```python
from build123d import *

# Parameters (mm, degrees)
SKETCH1_W           = 55.88
SKETCH1_H           = 45.72
BOSS_EXTRUDE1_DEPTH = 2.54
CUT_EXTRUDE1_REACH  = 4.54
SKETCH2_R           = 1.7
BOSS_EXTRUDE2_DEPTH = 2.21996
CUT_EXTRUDE2_DEPTH  = 2.21996
CUT_EXTRUDE3_REACH  = 6.76
SKETCH6_R           = 2.25
SKETCH7_W           = 7.62
SKETCH7_H           = 2.21996
CUT_EXTRUDE4_DEPTH  = 56.88
FILLET1_R           = 2.54


with BuildPart() as part:
    # Sketch1 → Boss-Extrude1 (new body)
    with BuildSketch(Plane(origin=(0, 0, 0), x_dir=(1, 0, 0), z_dir=(0, 1, 0))):
        with Locations((27.94, 22.86)):
            Rectangle(SKETCH1_W, SKETCH1_H)
    extrude(amount=BOSS_EXTRUDE1_DEPTH)

    # Sketch2 → Cut-Extrude1 (cut, up to next)
    with BuildSketch(Plane(origin=(0, 2.54, 0), x_dir=(1, 0, 0), z_dir=(0, 1, 0)), mode=Mode.PRIVATE) as cut_extrude1_sk1:
        with Locations((5.08, 40.64)):
            Circle(SKETCH2_R)
    cut_extrude1_tool1 = extrude(cut_extrude1_sk1.sketch, amount=-CUT_EXTRUDE1_REACH, mode=Mode.PRIVATE) & part.part
    add(cut_extrude1_tool1.solids().sort_by_distance((5.08, 2.54, -40.64))[0], mode=Mode.SUBTRACT)
    # Sketch2 → Cut-Extrude1 (cut, up to next)
    with BuildSketch(Plane(origin=(0, 2.54, 0), x_dir=(1, 0, 0), z_dir=(0, 1, 0)), mode=Mode.PRIVATE) as cut_extrude1_sk2:
        with Locations((50.8, 40.64)):
            Circle(SKETCH2_R)
    cut_extrude1_tool2 = extrude(cut_extrude1_sk2.sketch, amount=-CUT_EXTRUDE1_REACH, mode=Mode.PRIVATE) & part.part
    add(cut_extrude1_tool2.solids().sort_by_distance((50.8, 2.54, -40.64))[0], mode=Mode.SUBTRACT)
    # Sketch2 → Cut-Extrude1 (cut, up to next)
    with BuildSketch(Plane(origin=(0, 2.54, 0), x_dir=(1, 0, 0), z_dir=(0, 1, 0)), mode=Mode.PRIVATE) as cut_extrude1_sk3:
        with Locations((50.8, 5.08)):
            Circle(SKETCH2_R)
    cut_extrude1_tool3 = extrude(cut_extrude1_sk3.sketch, amount=-CUT_EXTRUDE1_REACH, mode=Mode.PRIVATE) & part.part
    add(cut_extrude1_tool3.solids().sort_by_distance((50.8, 2.54, -5.08))[0], mode=Mode.SUBTRACT)
    # Sketch2 → Cut-Extrude1 (cut, up to next)
    with BuildSketch(Plane(origin=(0, 2.54, 0), x_dir=(1, 0, 0), z_dir=(0, 1, 0)), mode=Mode.PRIVATE) as cut_extrude1_sk4:
        with Locations((5.08, 5.08)):
            Circle(SKETCH2_R)
    cut_extrude1_tool4 = extrude(cut_extrude1_sk4.sketch, amount=-CUT_EXTRUDE1_REACH, mode=Mode.PRIVATE) & part.part
    add(cut_extrude1_tool4.solids().sort_by_distance((5.08, 2.54, -5.08))[0], mode=Mode.SUBTRACT)

    # Sketch4 → Boss-Extrude2 (add)
    with BuildSketch(Plane(origin=(0, 2.54, 0), x_dir=(1, 0, 0), z_dir=(0, 1, 0))):
        Polygon((0, 30.48), (20.32, 45.72), (35.56, 45.72), (55.88, 30.48), (55.88, 15.24), (35.56, 0), (20.32, 0), (0, 15.24), align=None)
    extrude(amount=BOSS_EXTRUDE2_DEPTH)

    # Sketch5 → Cut-Extrude2 (cut)
    with BuildSketch(Plane.XZ):
        with BuildLine():
            Line((3.062941176, -18.986804383), (15.613529412, -8.335516435))
            ThreePointArc((15.613529412, -8.335516435), (27.94, -3.81), (40.266470588, -8.335516435))
            Line((40.266470588, -8.335516435), (52.817058824, -18.986804383))
            ThreePointArc((52.817058824, -18.986804383), (54.61, -22.86), (52.817058824, -26.733195617))
            Line((52.817058824, -26.733195617), (40.266470588, -37.384483565))
            ThreePointArc((40.266470588, -37.384483565), (27.94, -41.91), (15.613529412, -37.384483565))
            Line((15.613529412, -37.384483565), (3.062941176, -26.733195617))
            ThreePointArc((3.062941176, -26.733195617), (1.27, -22.86), (3.062941176, -18.986804383))
        make_face()
    extrude(amount=-CUT_EXTRUDE2_DEPTH, mode=Mode.SUBTRACT)

    # Sketch6 → Cut-Extrude3 (cut, up to next)
    with BuildSketch(Plane(origin=(0, 4.75996, 0), x_dir=(1, 0, 0), z_dir=(0, 1, 0)), mode=Mode.PRIVATE) as cut_extrude3_sk1:
        with Locations((6.35, 22.86)):
            Circle(SKETCH6_R)
    cut_extrude3_tool1 = extrude(cut_extrude3_sk1.sketch, amount=-CUT_EXTRUDE3_REACH, mode=Mode.PRIVATE) & part.part
    add(cut_extrude3_tool1.solids().sort_by_distance((6.35, 4.75996, -22.86))[0], mode=Mode.SUBTRACT)
    # Sketch6 → Cut-Extrude3 (cut, up to next)
    with BuildSketch(Plane(origin=(0, 4.75996, 0), x_dir=(1, 0, 0), z_dir=(0, 1, 0)), mode=Mode.PRIVATE) as cut_extrude3_sk2:
        with Locations((49.53, 22.86)):
            Circle(SKETCH6_R)
    cut_extrude3_tool2 = extrude(cut_extrude3_sk2.sketch, amount=-CUT_EXTRUDE3_REACH, mode=Mode.PRIVATE) & part.part
    add(cut_extrude3_tool2.solids().sort_by_distance((49.53, 4.75996, -22.86))[0], mode=Mode.SUBTRACT)

    # Sketch7 → Cut-Extrude4 (cut, through all)
    with BuildSketch(Plane.ZY):
        with Locations((-22.86, 1.10998)):
            Rectangle(SKETCH7_W, SKETCH7_H)
    extrude(amount=-CUT_EXTRUDE4_DEPTH, mode=Mode.SUBTRACT)

    # Fillet1
    fillet1_edges = [part.edges().sort_by_distance(p)[0] for p in [
        (0, 3.64998, -30.48),
        (0, 3.64998, -15.24),
        (20.32, 3.64998, 0),
        (35.56, 3.64998, 0),
        (55.88, 3.64998, -15.24),
        (55.88, 3.64998, -30.48),
        (35.56, 3.64998, -45.72),
        (20.32, 3.64998, -45.72),
    ]]
    fillet(fillet1_edges, radius=FILLET1_R)


solid = part.part
```
The listing builds one solid part. Answer for the finished solid, in the listing's coordinates (mm). A direction names the side the tool comes from. Coordinates: 2 decimals unless noted, no trailing zeros. Loops run counter-clockwise (first coordinate to the right, second up) from the corner with the lowest first, then second, coordinate; pieces in that order, holes last. Notation, with made-up numbers: (19, -1.5) -> (25, -1.5) arc R19 cw to (25, 30.5) -> close; hole circle Ø6 at (16, 61). An arc over 180 degrees is marked (long way). Return JSON: item names as keys, results as strings. Group by question number.
(1) A cutting plane is placed at A-A on y = 0.95. Write down the section's boundary in (x, z).
(2) A cutting plane is placed at B-B on z = -22.86. Write down the section's boundary in (x, y), and give its area (3 significant figures).
(3) Which of the six approach directions +Z, -Z, +X, -X, +Y, -Y give full straight-line access (tool end or side, diameter ignored) to faces 5 (the flat face through (50, 2.54, -7)), 6 (the flat face through (46.63, 1.094, -31.984)), 7 (the flat face through (8, 2.54, -41)), 8 (the flat face through (1, 1, -26.67)), 9 (the cylindrical face through (6.06, 3.51, -25.09))?
(4) Determine the mould class of faces 1 (the cylindrical face through (3.83, 1.29, -41.79)), 2 (the cylindrical face through (20.353, 3.666, -0.134)), 3 (the flat face through (48, 2.54, -41)), 4 (the flat face through (45.68, 3.63, -7.59)) for opening direction X: released by +X, released by -X, zero draft, split by the parting line, or undercut.
(5) Given pin 1 Ø4 at (x, z) = (5.08, -5.08) entering from +Y; pin 2 Ø5 at (x, z) = (6.35, -22.86) entering from -Y; pin 3 Ø2 at (x, z) = (50.8, -5.08) entering from +Y, each flat-ended and moving along its own axis, determine where each tip first touches the part or whether it passes through.
(6) Find the intervals of material crossed by probe 1 along X at (y, z) = (2.9, -22.86); probe 2 along Z at (x, y) = (5.08, 1.9) (3 decimals); probe 3 along X at (y, z) = (1, -40), in increasing order. Write a range as from..to.
(7) A cutting plane is placed at D-D on y = 3.7. Write down the section's boundary in (x, z).
(8) A cutting plane is placed at C-C on x = 5.08. Write down the section's boundary in (y, z) (3 decimals).
The answers:
{
 "1": {"outline": "(0, -45.72) -> (55.88, -45.72) -> (55.88, -26.67) -> (52.89, -26.67) arc R5.08 cw to (52.82, -26.73) -> (40.27, -37.38) arc R19.05 cw to (15.61, -37.38) -> (3.06, -26.73) arc R5.08 cw to (2.99, -26.67) -> (0, -26.67) -> close; (0, -19.05) -> (2.99, -19.05) arc R5.08 cw to (3.06, -18.99) -> (15.61, -8.34) arc R19.05 cw to (40.27, -8.34) -> (52.82, -18.99) arc R5.08 cw to (52.89, -19.05) -> (55.88, -19.05) -> (55.88, 0) -> (0, 0) -> close; hole circle Ø3.4 at (5.08, -40.64); hole circle Ø3.4 at (5.08, -5.08); hole circle Ø3.4 at (50.8, -40.64); hole circle Ø3.4 at (50.8, -5.08)"},
 "2": {"outline": "(0, 2.22) -> (4.1, 2.22) -> (4.1, 4.76) -> (0, 4.76) -> close; (8.6, 2.22) -> (47.28, 2.22) -> (47.28, 4.76) -> (8.6, 4.76) -> close; (51.78, 2.22) -> (55.88, 2.22) -> (55.88, 4.76) -> (51.78, 4.76) -> close", "area": "119 mm^2"},
 "3": {"face 5": "+Z, +X, +Y", "face 6": "-Y", "face 7": "-Z, -X, +Y", "face 8": "+X, -X, -Y", "face 9": "+Y, -Y"},
 "4": {"face 1": "undercut", "face 2": "released by -X", "face 3": "zero draft", "face 4": "released by +X"},
 "5": {"pin 1": "stops at y = 2.54", "pin 2": "stops at y = 2.22", "pin 3": "passes through"},
 "6": {"probe 1": "x = 0..4.1, 8.6..47.28, 51.78..55.88", "probe 2": "z = -45.72..-42.34, -38.94..-28.445, -17.275..-6.78, -3.38..0", "probe 3": "x = 0..3.51, 6.65..19.63, 36.25..49.23, 52.37..55.88"},
 "7": {"outline": "(0, -29.21) arc R2.54 ccw to (1.02, -31.24) -> (19.64, -45.21) arc R2.54 ccw to (21.17, -45.72) -> (34.71, -45.72) arc R2.54 ccw to (36.24, -45.21) -> (54.86, -31.24) arc R2.54 ccw to (55.88, -29.21) -> (55.88, -16.51) arc R2.54 ccw to (54.86, -14.48) -> (36.24, -0.51) arc R2.54 ccw to (34.71, 0) -> (21.17, 0) arc R2.54 ccw to (19.64, -0.51) -> (1.02, -14.48) arc R2.54 ccw to (0, -16.51) -> close; hole circle Ø4.5 at (6.35, -22.86); hole circle Ø4.5 at (49.53, -22.86)"},
 "8": {"outline": "(0, -45.72) -> (2.54, -45.72) -> (2.54, -42.34) -> (0, -42.34) -> close; (0, -38.94) -> (2.54, -38.94) -> (2.54, -34.29) -> (4.76, -34.29) -> (4.76, -24.717) -> (2.22, -24.717) -> (2.22, -28.445) -> (0, -28.445) -> close; (0, -17.275) -> (2.22, -17.275) -> (2.22, -21.003) -> (4.76, -21.003) -> (4.76, -11.43) -> (2.54, -11.43) -> (2.54, -6.78) -> (0, -6.78) -> close; (0, -3.38) -> (2.54, -3.38) -> (2.54, 0) -> (0, 0) -> close"}
}
